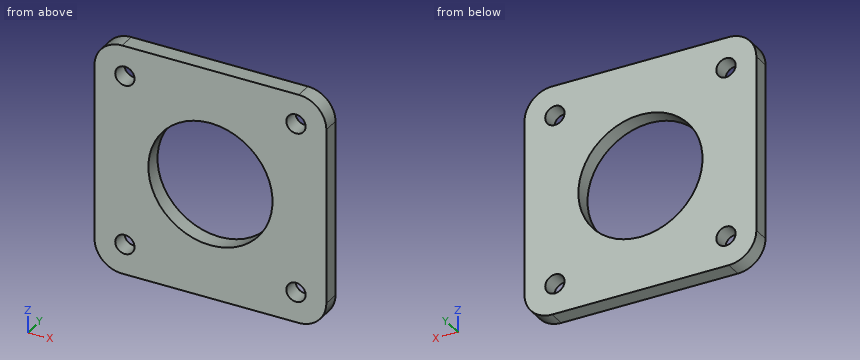
from build123d import *

# Parameters (mm, degrees)
SKETCH1_W           = 42
SKETCH1_H           = 42
BOSS_EXTRUDE1_DEPTH = 3
SKETCH2_R           = 1.75
SKETCH2_R_2         = 11.25
CUT_EXTRUDE1_DEPTH  = 30.849623113
FILLET1_R           = 5


with BuildPart() as part:
    # Sketch1 → Boss-Extrude1 (new body)
    with BuildSketch(Plane(origin=(0, 0, 0), x_dir=(1, 0, 0), z_dir=(0, 1, 0))):
        Rectangle(SKETCH1_W, SKETCH1_H)
    extrude(amount=BOSS_EXTRUDE1_DEPTH)

    # Sketch2 → Cut-Extrude1 (cut, through all)
    with BuildSketch(Plane(origin=(0, 3, 0), x_dir=(1, 0, 0), z_dir=(0, 1, 0))):
        with Locations(Location((-15.5, 15.5, 0), (0, 0, 270))):
            Circle(SKETCH2_R)
        with Locations(Location((15.5, 15.5, 0), (0, 0, 270))):
            Circle(SKETCH2_R)
        with Locations(Location((15.5, -15.5, 0), (0, 0, 270))):
            Circle(SKETCH2_R)
        with Locations(Location((-15.5, -15.5, 0), (0, 0, 270))):
            Circle(SKETCH2_R)
        with Locations(Location((0, 0, 0), (0, 0, 270))):
            Circle(SKETCH2_R_2)
    extrude(amount=-CUT_EXTRUDE1_DEPTH, mode=Mode.SUBTRACT)

    # Fillet1
    fillet1_edges = [part.edges().sort_by_distance(p)[0] for p in [
        (21, 1.5, 21),
        (-21, 1.5, 21),
        (-21, 1.5, -21),
        (21, 1.5, -21),
    ]]
    fillet(fillet1_edges, radius=FILLET1_R)


solid = part.part
Source: CAD feature listing. Evaluate the final solid. Frame: model axes, mm. Coordinates: 2 decimals unless noted, no trailing zeros. Loops run counter-clockwise (first coordinate to the right, second up) from the corner with the lowest first, then second, coordinate; pieces in that order, holes last. Notation, with made-up numbers: M 24.5,70 L 81.5,70 A33 ccw 81.5,100 Z; hole C 30,-39.75 d10. An arc over 180 degrees is marked long. Answer in a Markdown table with one row per item.
Q1. Section A-A on x = -15.5. Return the cut outline in (y, z), plus the area to 3 significant figures.
Answers below:
| item | result |
|---|---|
| outline | M 0,-21 L 3,-21 L 3,-17.25 L 0,-17.25 Z; M 0,-13.75 L 3,-13.75 L 3,13.75 L 0,13.75 Z; M 0,17.25 L 3,17.25 L 3,21 L 0,21 Z |
| area | 105 mm^2 |
Q2. Section D-D on z = -15.5. Return the cut outline in (x, y).
Answers below:
| item | result |
|---|---|
| outline | M -21,0 L -17.25,0 L -17.25,3 L -21,3 Z; M -13.75,0 L 13.75,0 L 13.75,3 L -13.75,3 Z; M 17.25,0 L 21,0 L 21,3 L 17.25,3 Z |
Q3. Section C-C on y = 0.65. Return the cut outline in (x, z).
Answers below:
| item | result |
|---|---|
| outline | M -21,-16 A5 ccw -16,-21 L 16,-21 A5 ccw 21,-16 L 21,16 A5 ccw 16,21 L -16,21 A5 ccw -21,16 Z; hole C -15.5,-15.5 d3.5; hole C -15.5,15.5 d3.5; hole C 0,0 d22.5; hole C 15.5,-15.5 d3.5; hole C 15.5,15.5 d3.5 |
Q4. Ray query, probe 1 along X at (y, z) = (1.1, -15.5); probe 2 along X at (y, z) = (1.45, 0); probe 3 along X at (y, z) = (1.1, 17). Return the intervals inside material, ascending. Write a range as from..to.
Answers below:
| item | result |
|---|---|
| probe 1 | x = -21..-17.25, -13.75..13.75, 17.25..21 |
| probe 2 | x = -21..-11.25, 11.25..21 |
| probe 3 | x = -20.9..-16.4, -14.6..14.6, 16.4..20.9 |
Q5. Section B-B on z = 0. Return the cut outline in (x, y).
Answers below:
| item | result |
|---|---|
| outline | M -21,0 L -11.25,0 L -11.25,3 L -21,3 Z; M 11.25,0 L 21,0 L 21,3 L 11.25,3 Z |
